Autodesk Inventor part; units mm, degrees
ref_plane "YZ Plane" through (0, 0, 0) normal (1, 0, 0) x (0, 1, 0)
ref_plane "XZ Plane" through (0, 0, 0) normal (0, 1, 0) x (-1, 0, 0)
ref_plane "XY Plane" through (0, 0, 0) normal (0, 0, 1) x (1, 0, 0)
ref_plane "РабПлоскость2" through (0, 0, 5) normal (0, 0, 1) x (1, 0, 0)
sketch "Эскиз1" plane through (0, 0, 5) normal (0, 0, 1) x (1, 0, 0)
  line L0 (-14.2362, -16) -> (14.1136, -16)
  arc A0 (14.1136, -15.5263) -> (14.1136, -16) centre (14.9819, -15.7632) ccw
  line L1 (-14.2362, 16) -> (-14.2362, -16)
  line L2 (-18.2362, 20) -> (18.2362, 20)
  line L3 (18.2362, 20) -> (18.2362, -20)
  line L4 (18.2362, -20) -> (-18.2362, -20)
  line L5 (-18.2362, -20) -> (-18.2362, 20)
  circle A1 centre (9.2362, 0) radius 1.6
  circle A2 centre (-9.2362, 0) radius 1.6
  circle A3 centre (0.7638, 0) radius 2.15
  circle A4 centre (19.2362, 0) radius 2.15
  line L6 (14.1136, -15.5263) -> (14.1136, -16)
  line L7 (14.1136, -16) -> (23.5645, -16)
  line L8 (23.5645, -16) -> (23.5645, 16)
  line L9 (23.5645, 16) -> (-14.2362, 16)
  circle A5 centre (9.2362, -11) radius 3.25
  circle A6 centre (9.2362, 11) radius 3.25
  circle A7 centre (-9.2362, -11) radius 3.25
  circle A8 centre (-9.2362, 11) radius 3.25
  point P0 (14.2362, 16)
  dimension "d0" = 4
  dimension "d2" = 4
extrude "Выдавливание1" add sketch "Эскиз1" along normal blind 3 contours A0 L6 | L1 L9 L3 A4 L7 L0 | L0 L7 L3 L4 L5 L2 L9 L1 | A4 L3 | A1 | A2 | A3 | A5 | A6 | A7 | A8 picked at (17.8581, 0.0863)
sketch "Эскиз3" plane through (-18.2362, 20, 5) normal (0, 1, 0) x (1, 0, 0)
  line L0 (0, -3) -> (36.4725, -3)
  line L1 (36.4725, -3) -> (36.4725, -18.4215)
  line L2 (36.4725, -18.4215) -> (18.2361, -3)
  line L3 (18.2361, -3) -> (0, -18.4219)
  line L4 (0, -18.4219) -> (0, -3)
  point P0 (18.2362, 5)
  point P1 (18.2361, -3)
  point P2 (18.2361, -3)
extrude "Выдавливание2" add sketch "Эскиз3" against normal up to surface (40 mm away)
ref_plane "РабПлоскость4" through (0, 0, 8) normal (0, 0, 1) x (1, 0, 0)
sketch "Эскиз4" plane through (0, 0, 8) normal (0, 0, 1) x (1, 0, 0)
  circle A0 centre (9.2362, 0) radius 1.6
  circle A1 centre (-9.2362, 0) radius 1.6
  circle A2 centre (9.2362, 0) radius 2.7434
  circle A3 centre (-9.2362, 0) radius 2.7434
  point P0 (0, 0)
extrude "Выдавливание3" cut sketch "Эскиз4" along normal blind 14.75 contours A0 | A1 | A2 | A3
sketch "Эскиз5" plane through (0, 0, 5) normal (0, 0, -1) x (-1, 0, 0)
  line L0 (18.2362, 20) -> (18.2362, -20)
  line L1 (18.2362, 20) -> (23.2362, 20)
  line L2 (23.2362, 20) -> (23.2362, -20)
  line L3 (23.2362, -20) -> (18.2362, -20)
  line L4 (18.2362, -20) -> (18.2362, 20)
  line L5 (0.0002, -20) -> (-18.2362, -20)
  line L6 (-18.2362, -20) -> (-23.2362, -20)
  line L7 (-23.2362, -20) -> (-23.2362, 20)
  line L8 (-23.2362, 20) -> (-18.2362, 20)
  line L9 (-18.2362, 20) -> (-18.2362, -20)
  point P0 (0, 0)
  dimension "d11" = 5
  dimension "d12" = 5
extrude "Выдавливание4" add sketch "Эскиз5" against normal blind 30
sketch "Эскиз6" plane through (0, 0, 35) normal (0, 0, 1) x (1, 0, 0)
  line L0 (-23.2362, 20) -> (23.2362, 20)
  line L1 (23.2362, 20) -> (23.2362, -20)
  line L2 (23.2362, -20) -> (-23.2362, -20)
  line L3 (-23.2362, -20) -> (-23.2362, 20)
  circle A0 centre (0, 0) radius 1.55
  line L4 (23.2362, -20) -> (23.2362, 20)
  line L5 (23.2362, 20) -> (18.2362, 20)
  line L6 (-23.2362, 20) -> (-23.2362, -20)
  line L7 (-0.0002, -20) -> (18.2362, -20)
  dimension "d15" = 3.1
extrude "Выдавливание5" add sketch "Эскиз6" along normal blind 3
sketch "Эскиз7" plane through (0, 0, 38) normal (0, 0, 1) x (1, 0, 0)
  circle A0 centre (-9.2362, 0) radius 2.7434
  line L0 (-18.2362, -20) -> (-0.0002, -20)
  line L1 (-0.0002, 20) -> (-0.0002, -20)
  line L2 (-18.2362, 20) -> (-0.0002, 20)
  line L3 (-18.2362, 20) -> (-18.2362, -20)
  circle A1 centre (9.2362, 0) radius 2.7434
  line L4 (-0.0002, -20) -> (18.2362, -20)
  line L5 (18.2362, 20) -> (18.2362, -20)
  line L6 (-0.0002, 20) -> (18.2362, 20)
  line L7 (-0.0002, 20) -> (-0.0002, -20)
  circle A2 centre (-9.2362, 0) radius 4.6972
  circle A3 centre (9.2362, 0) radius 4.6972
  point P0 (0, 0)
extrude "Выдавливание6" cut sketch "Эскиз7" against normal up to surface (3 mm away) contours A0 | A1 | A2 | A3
properties part number "верх крепления маркера"
Check sheet for the modelled part. Datum: model origin and axes. Units: mm. A direction names the side the tool comes from. Give positions to 0.01 mm unless a question says otherwise; leave off trailing zeros. Order: outer loops, then holes, each group sorted by start corner. A loop starts at its lowest first (then second) coordinate and runs counter-clockwise, first axis right, second up. Notation, with made-up numbers: (-0.5, -33.75) - (34.5, -33.75) arc R10 cw to (34.5, -20.75) - close; hole circle Ø2 at (-14, 44.25). An arc over 180 degrees is marked (long way). Answer as CSV lines item,"result".
1. Section check D-D (z = 10). Record the boundary of the cut face in (x, y), then the cut area to 3 significant figures.
Result sheet:
outline,"(-23.24, -20) - (-2.37, -20) - (-2.37, 20) - (-23.24, 20) - close; (2.36, -20) - (23.24, -20) - (23.24, 20) - (2.36, 20) - close; hole circle Ø5.49 at (-9.24, 0); hole circle Ø5.49 at (9.24, 0)"
area,"1,620 mm²"
2. Go/stop test with flat-tipped pins: P1, Ø7, axis at x = 9.24, y = 0, coming from the +Z side; P2, Ø1.6, axis at x = 9, y = 0.5, coming from the +Z side. Record where each tip stops, or that it passes through.
Result sheet:
P1,"z = 18.77"
P2,"z = 8"
3. Section check C-C (x = -15). Record the boundary of the cut face in (y, z).
Result sheet:
outline,"(-20, 5) - (20, 5) - (20, 20.69) - (-20, 20.69) - close; (-20, 35) - (20, 35) - (20, 38) - (-20, 38) - close"
4. Scan lines: probe 1 along Z at (x, y) = (18, 16.5); probe 2 along X at (y, z) = (-2, 34); probe 3 along X at (y, z) = (0, 15). Record each from-to range of solid material in increasing order. Write a range as from..to.
Result sheet:
probe 1,"5..23.22, 35..38"
probe 2,"-23.24..-18.24, 18.24..23.24"
probe 3,"-23.24..-11.98, 11.98..23.24"
5. Mould release check, pull along X, two halves, no side actions. Record for faces 1 (the face through (0.715, 1.375, 36.479)), 2 (the face through (23.236, 0, 21)), 3 (the face through (-5, 20, 10)): released by +X, released by -X, zero draft, split by the parting line, or undercut.
Result sheet:
face 1,"undercut"
face 2,"released by +X"
face 3,"zero draft"
6. Section check B-B (y = -5.5). Record the boundary of the cut face in (x, z).
Result sheet:
outline,"(-23.24, 5) - (23.24, 5) - (23.24, 38) - (-23.24, 38) - close; hole (-18.24, 23.42) - (0, 8) - (18.24, 23.42) - (18.24, 35) - (-18.24, 35) - close"
7. Section check A-A (z = 26.5). Record the boundary of the cut face in (x, y), then the cut area to 3 significant figures.
Result sheet:
outline,"(-23.24, -20) - (-18.24, -20) - (-18.24, 20) - (-23.24, 20) - close; (18.24, -20) - (23.24, -20) - (23.24, 20) - (18.24, 20) - close"
area,"400 mm²"
8. Tool access check on faces 4 (the face through (-9, 0, 8)), 5 (the face through (0, 0, 5)), 6 (the face through (-8.99, 4.72, 15.6)). Record the directions out of +Z, -Z, +X, -X, +Y, -Y that give a thin tool (end or side, any length) a straight path to the whole face; none if there is none.
Result sheet:
face 4,"+Z"
face 5,"-Z, +X, -X, +Y, -Y"
face 6,"+Y, -Y"
